Check sheet for the drawn part. Datum: minimum x, y, z corner. Units: mm. Coordinates: 2 decimals unless noted, no trailing zeros. Loops run counter-clockwise (first coordinate to the right, second up) from the corner with the lowest first, then second, coordinate; pieces in that order, holes last.
Q1. Sectioned sample at A-A (y = 10.5). Enter the section's corners in (x, z), then the cut area to 3 significant figures.
Q2. Mould release check, pull along Y, two halves, no side actions. Record for the marked faces 1, 2, 3 and 4: +Y half, -Y half, draft (parallel to the pull), parting line (faces both ways), or undercut.
Q3. Material ranges on probe 1 along X at (y, z) = (10.5, 0.4); probe 2 along X at (y, z) = (7, 1.3), recorded low to high.
Q4. Sectioned sample at C-C (z = 1.2). Enter the section's corners in (x, y), then the cut area to 3 significant figures.
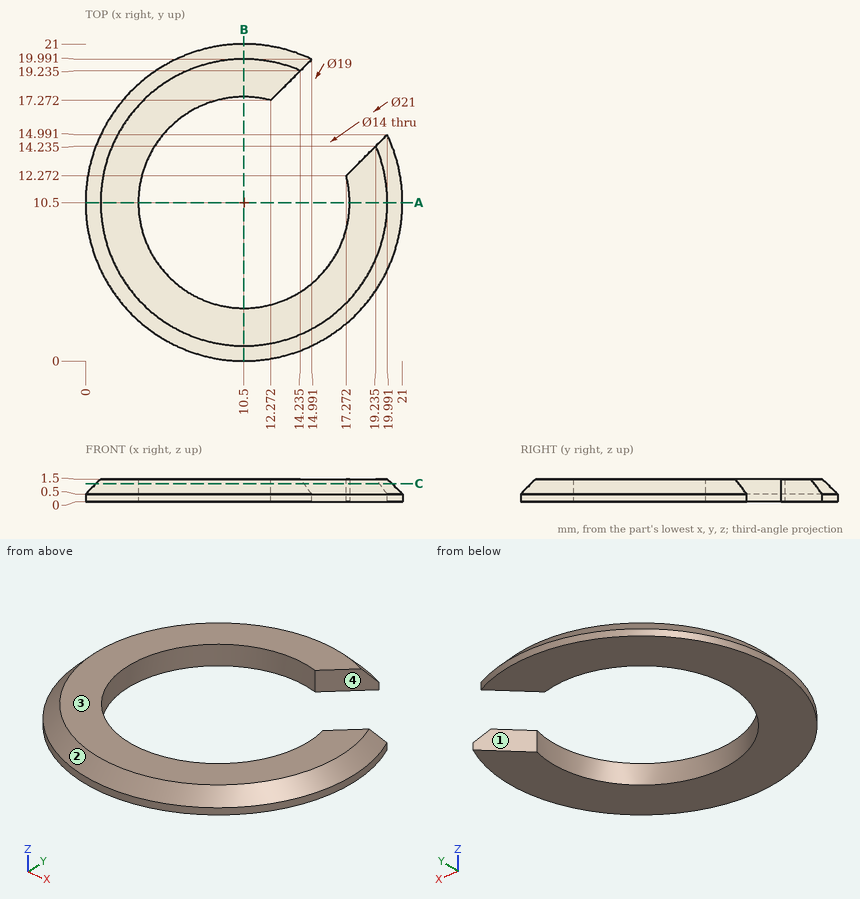
Geometry check:
1. outline: (0, 0) - (3.5, 0) - (3.5, 1.5) - (1, 1.5) - (0, 0.5) - close; (17.5, 0) - (21, 0) - (21, 0.5) - (20, 1.5) - (17.5, 1.5) - close
1. area: 9.50 mm2
2. face 1: +Y half
2. face 2: parting line
2. face 3: draft
2. face 4: undercut
3. probe 1: x = 0 to 3.5, 17.5 to 21
3. probe 2: x = 1.45 to 4.44, 16.56 to 19.55
4. outline: (12.27, 17.27) - (14.46, 19.46) arc R9.8 ccw (long way) to (19.46, 14.46) - (17.27, 12.27) arc R7 cw (long way) to start
4. area: 127 mm2
